Read the model definition and answer for the solid it produces. Units are mm, in the model's axes. A direction names the side the tool comes from. Coordinates: 2 decimals unless noted, no trailing zeros. Write each loop counter-clockwise with the first axis right and the second up, starting at its lowest first coordinate (ties: lowest second). Pieces come first, ordered by that corner, then holes. Notation, with made-up numbers: (44, 34.5) -> (80, 34.5) arc R24 ccw to (80, 62.5) -> close; hole circle Ø9 at (28, -2.5). An arc over 180 degrees is marked (long way). Write item = value, one per line. Start each with the question number.
1) A tool of negligible diameter and unlimited length cuts with its end or side. For faces 4 (the face through (1, 3, -4)), 5 (the face through (3, 1, -4)), 6 (the face through (3, 3, -8)), 7 (the face through (5, 3, -4)), from which of +Z, -Z, +X, -X, +Y, -Y can it reach the whole face along a straight path? Write none if from no direction.
2) Section D-D (z = 0.5) is taken. Determine the outline of the cut face in (x, y), plus the area to 3 significant figures.
3) Flat-ended cylindrical pins translate along their axes: pin 1 Ø4.5 at (y, z) = (2, -6.5) entering from +X; pin 2 Ø0.6 at (y, z) = (-1, 13) entering from -X; pin 3 Ø2 at (x, z) = (2.5, -3.5) entering from -Y. Find the tip coordinate at first contact, or state that the pin passes through.
4) Section B-B (y = 3) is taken. Determine the outline of the cut face in (x, z).
5) Section A-A (z = 13) is taken. Determine the outline of the cut face in (x, y).
6) Section C-C (x = 3) is taken. Determine the outline of the cut face in (y, z).
7) Find the intervals of material crossed by line 1 along Y through (x, z) = (3, -8.25); line 2 along X through (y, z) = (3, -8.25); line 3 along Z through (x, y) = (2.4, 2.5), in increasing order. Write a range as from..to.
8) For a pull along X with two mould halves and no side action, classify faces 1 (the face through (3, 3, 26)), 2 (the face through (3, 4.5, -7)), 3 (the face through (3.54, 0.56, 22.96)) as released by +X, released by -X, zero draft, split by the parting line, or undercut.
Autodesk Fusion 360 part; units mm, degrees
sketch "草图1" plane through (0, 0, 0) normal (0, 0, 1) x (1, 0, 0)
  line L0 (0, 0) -> (6, 0)
  line L1 (6, 0) -> (6, 6)
  line L2 (6, 6) -> (0, 6)
  line L3 (0, 6) -> (0, 0)
extrude "拉伸1" add sketch "草图1" along normal blind 20
sketch "草图2" plane through (0, 0, 0) normal (0, -1, 0) x (1, 0, 0)
  line L0 (0, 0) -> (6, 0)
  line L1 (6, 0) -> (6, 20)
  line L2 (6, 20) -> (0, 20)
  line L3 (0, 20) -> (0, 0)
  line L4 (0, 20) -> (1.5, 20)
  line L5 (1.5, 20) -> (1.5, 10)
  line L6 (1.5, 10) -> (0, 10)
  line L7 (0, 10) -> (0, 20)
  line L8 (0, 10) -> (0, 20)
  line L9 (0, 20) -> (1.5, 20)
  line L10 (1.5, 20) -> (1.5, 10)
  line L11 (0, 10) -> (0, 20)
  line L12 (1.5, 10) -> (0, 10)
  line L13 (0, 10) -> (0, 20)
  line L14 (0, 10) -> (0, 20)
  line L15 (1.5, 20) -> (1.5, 10)
  line L16 (0, 10) -> (0, 20)
  line L17 (0, 20) -> (1.5, 20)
  line L18 (1.5, 20) -> (1.5, 10)
  line L19 (1.5, 10) -> (0, 10)
  line L20 (0, 10) -> (0, 20)
  line L21 (1.5, 10) -> (0, 10)
  line L22 (0, 20) -> (1.5, 20)
  line L23 (0, 10) -> (0, 20)
  line L24 (4.4997, 10.0138) -> (4.4997, 20.0138)
  line L25 (5.9997, 20.0138) -> (5.9997, 10.0138)
  line L26 (4.4997, 10.0138) -> (4.4997, 20.0138)
  line L27 (4.4997, 20.0138) -> (5.9997, 20.0138)
  line L28 (5.9997, 20.0007) -> (5.9997, 10.0007)
  line L29 (5.9997, 10.0138) -> (4.4997, 10.0138)
  line L30 (4.4997, 10.0007) -> (4.4997, 20.0007)
  line L31 (5.9997, 10.0007) -> (4.4997, 10.0007)
  line L32 (4.4997, 20.0007) -> (5.9997, 20.0007)
  line L33 (4.4997, 10.0138) -> (4.4997, 20.0138)
  line L34 (1.5, 20) -> (4.4997, 20)
  line L35 (4.4997, 20) -> (4.4997, 10)
  line L36 (4.4997, 10) -> (1.5, 10)
  line L37 (1.5, 10) -> (1.5, 20)
  point P0 (0, 20)
  point P1 (0, 20)
  point P2 (0, 20)
  point P3 (4.4997, 20.0138)
  point P4 (4.4997, 20.0007)
  dimension "d3" = 10
  dimension "d4" = 10
  dimension "d5" = 10
  dimension "d6" = 10
  dimension "d7" = 10
  dimension "d8" = 10
  dimension "d9" = 10
  dimension "d10" = 10
  dimension "d11" = 10
  dimension "d12" = 10
  dimension "d13" = 10
  dimension "d14" = 10
  dimension "d15" = 10
extrude "拉伸2" add sketch "草图2" along normal blind 2 contours L2 L5 L10 L15 L18 L24 L26 L30 L33 L34 L35 L36 L37
sketch "草图3" plane through (0, 0, 20) normal (0, 0, 1) x (-1, 0, 0)
  line L0 (0, -6) -> (0, 0)
  line L1 (0, 0) -> (-1.5, 0)
  line L2 (-1.5, 0) -> (-1.5, 2)
  line L3 (-1.5, 2) -> (-4.4997, 2)
  line L4 (-4.4997, 2) -> (-4.4997, 0)
  line L5 (-4.4997, 0) -> (-6, 0)
  line L6 (-6, 0) -> (-6, -6)
  line L7 (-6, -6) -> (0, -6)
  circle A0 centre (-3, -3) radius 2.5
  dimension "d18" = 5
extrude "拉伸3" add sketch "草图3" along normal blind 6 contours A0
sketch "草图4" plane through (0, 0, 0) normal (0, 0, -1) x (1, 0, 0)
  line L0 (0, 0) -> (0, -6)
  line L1 (0, -6) -> (6, -6)
  line L2 (6, -6) -> (6, 0)
  line L3 (6, 0) -> (0, 0)
  line L4 (0, 0) -> (1, 0)
  line L5 (1, 0) -> (1, -6)
  line L6 (1, -6) -> (0, -6)
  line L7 (0, -6) -> (0, 0)
  line L8 (5, 0) -> (6, 0)
  line L9 (6, 0) -> (6, -6)
  line L10 (6, -6) -> (5, -6)
  line L11 (5, -6) -> (5, 0)
  line L12 (6, -5) -> (0, -5)
  line L13 (0, -5) -> (0, -6)
  line L14 (0, -6) -> (6, -6)
  line L15 (6, -6) -> (6, -5)
  line L16 (0, 0) -> (6, 0)
  line L17 (6, 0) -> (6, -1)
  line L18 (6, -1) -> (0, -1)
  line L19 (0, -1) -> (0, 0)
  line L20 (1, -1) -> (5, -1)
  line L21 (5, -1) -> (5, -5)
  line L22 (5, -5) -> (1, -5)
  line L23 (1, -5) -> (1, -1)
extrude "拉伸4" add sketch "草图4" along normal blind 6 contours L5 L11 L12 L18 L20 L21 L22 L23
sketch "草图5" plane through (0, 0, -6) normal (0, 0, -1) x (1, 0, 0)
  line L0 (5, -5) -> (5, -1)
  line L1 (5, -1) -> (1, -1)
  line L2 (1, -1) -> (1, -5)
  line L3 (1, -1) -> (5, -1)
  line L4 (5, -1) -> (5, -5)
  line L5 (1, -5) -> (1, -1)
  line L6 (1, -5) -> (2, -5)
  line L7 (2, -5) -> (2, -4.5)
  line L8 (2, -4.5) -> (4, -4.5)
  line L9 (4, -4.5) -> (4, -5)
  line L10 (4, -5) -> (5, -5)
  circle A0 centre (3, -3) radius 1
  dimension "d23" = 2
extrude "拉伸5" add sketch "草图5" along normal blind 3 contours L0 L1 L2 L3 L4 L5 L6 L7 L8 L9 L10 | A0
sketch "草图6" plane through (0, 0, -9) normal (0, 0, -1) x (1, 0, 0)
  line L0 (1, -5) -> (2, -5)
  line L1 (2, -5) -> (2, -4.5)
  line L2 (2, -4.5) -> (4, -4.5)
  line L3 (4, -4.5) -> (4, -5)
  line L4 (4, -5) -> (5, -5)
  line L5 (5, -5) -> (5, -1)
  line L6 (5, -1) -> (1, -1)
  line L7 (1, -1) -> (1, -5)
  circle A0 centre (3, -3) radius 1
  dimension "d26" = 2
extrude "拉伸6" cut sketch "草图6" against normal blind 1 contours A0
Answer key:
q1.face_4 = -Z, -X, +Y, -Y
q1.face_5 = -Z, +X, -X, -Y
q1.face_6 = -Z
q1.face_7 = -Z, +X, +Y, -Y
q2.outline = (0, 0) -> (6, 0) -> (6, 6) -> (0, 6) -> close
q2.area = 36.0 mm^2
q3.pin_1 = 5
q3.pin_2 = 1.5
q3.pin_3 = 1
q4.outline = (0, 0) -> (1, 0) -> (1, -9) -> (2, -9) -> (2, -8) -> (4, -8) -> (4, -9) -> (5, -9) -> (5, 0) -> (6, 0) -> (6, 20) -> (5.5, 20) -> (5.5, 26) -> (0.5, 26) -> (0.5, 20) -> (0, 20) -> close
q5.outline = (0, 0) -> (1.5, 0) -> (1.5, -2) -> (4.5, -2) -> (4.5, 0) -> (6, 0) -> (6, 6) -> (0, 6) -> close
q6.outline = (-2, 10) -> (0, 10) -> (0, 0) -> (1, 0) -> (1, -9) -> (2, -9) -> (2, -8) -> (4, -8) -> (4, -9) -> (4.5, -9) -> (4.5, -6) -> (5, -6) -> (5, 0) -> (6, 0) -> (6, 20) -> (5.5, 20) -> (5.5, 26) -> (0.5, 26) -> (0.5, 20) -> (-2, 20) -> close
q7.line_1 = 1..2, 4..4.5
q7.line_2 = 1..2, 4..5
q7.line_3 = -8..26
q8.face_1 = zero draft
q8.face_2 = undercut
q8.face_3 = split by the parting line
